The listing builds one solid part. Answer for the finished solid, in the listing's coordinates (mm). Give positions to 0.01 mm unless a question says otherwise; leave off trailing zeros. Order: outer loops, then holes, each group sorted by start corner. A loop starts at its lowest first (then second) coordinate and runs counter-clockwise, first axis right, second up. Notation, with made-up numbers: (50.5, 7) -> (95.5, 7) arc R25 ccw to (95.5, 38) -> close; hole circle Ø1 at (-16.5, 84). An arc over 180 degrees is marked (long way). Answer as a JSON object with one key per item and string values. Group by question number.
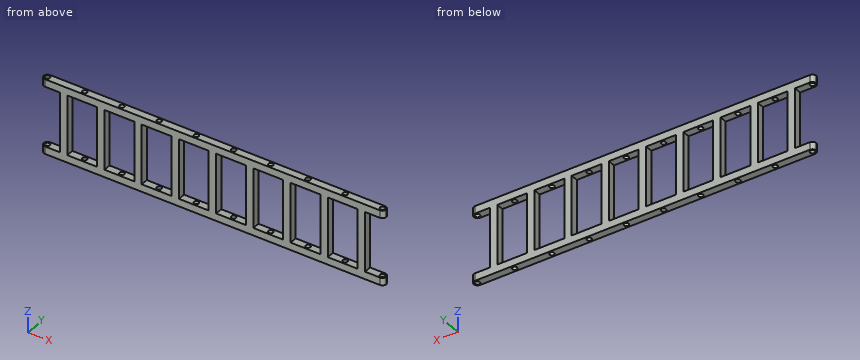
```python
from build123d import *

# Parameters (mm, degrees)
SKETCH1_W           = 25.4
SKETCH1_H           = 50.8
BOSS_EXTRUDE1_DEPTH = 6.35
CUT_EXTRUDE1_REACH  = 161.384
SKETCH2_R           = 1.9939
FILLET2_R           = 3.175


with BuildPart() as part:
    # Sketch1 → Boss-Extrude1 (new body)
    with BuildSketch(Plane(origin=(0, 0, 0), x_dir=(1, 0, 0), z_dir=(0, 1, 0))):
        Polygon((-146.05, 25.4), (-130.175, 25.4), (-130.175, -25.4), (-146.05, -25.4), (-146.05, -31.75), (146.05, -31.75), (146.05, -25.4), (130.175, -25.4), (130.175, 25.4), (146.05, 25.4), (146.05, 31.75), (-146.05, 31.75), align=None)
        with Locations((-15.875, 0)):
            Rectangle(SKETCH1_W, SKETCH1_H, mode=Mode.SUBTRACT)
        with Locations((111.125, 0)):
            Rectangle(SKETCH1_W, SKETCH1_H, mode=Mode.SUBTRACT)
        with Locations((-47.625, 0)):
            Rectangle(SKETCH1_W, SKETCH1_H, mode=Mode.SUBTRACT)
        with Locations((-79.375, 0)):
            Rectangle(SKETCH1_W, SKETCH1_H, mode=Mode.SUBTRACT)
        with Locations((-111.125, 0)):
            Rectangle(SKETCH1_W, SKETCH1_H, mode=Mode.SUBTRACT)
        with Locations((79.375, 0)):
            Rectangle(SKETCH1_W, SKETCH1_H, mode=Mode.SUBTRACT)
        with Locations((47.625, 0)):
            Rectangle(SKETCH1_W, SKETCH1_H, mode=Mode.SUBTRACT)
        with Locations((15.875, 0)):
            Rectangle(SKETCH1_W, SKETCH1_H, mode=Mode.SUBTRACT)
    extrude(amount=-BOSS_EXTRUDE1_DEPTH)

    # Cut-Extrude1: up to this face of the body (flat: up to its plane)
    cut_extrude1_end = Plane(part.part.faces().sort_by_distance((0, -3.175, -31.75))[0])
    # Sketch2 → Cut-Extrude1 (cut, up to the picked face)
    with BuildSketch(Plane.XY.offset(31.75), mode=Mode.PRIVATE) as cut_extrude1_sk1:
        with Locations((-142.875, -3.175)):
            Circle(SKETCH2_R)
    cut_extrude1_tool1 = split(extrude(cut_extrude1_sk1.sketch, amount=-CUT_EXTRUDE1_REACH, mode=Mode.PRIVATE), bisect_by=cut_extrude1_end, keep=Keep.BOTH, mode=Mode.PRIVATE)
    # Sketch2 → Cut-Extrude1 (cut, up to the picked face)
    with BuildSketch(Plane.XY.offset(31.75), mode=Mode.PRIVATE) as cut_extrude1_sk2:
        with Locations((-111.125, -3.175)):
            Circle(SKETCH2_R)
    cut_extrude1_tool2 = split(extrude(cut_extrude1_sk2.sketch, amount=-CUT_EXTRUDE1_REACH, mode=Mode.PRIVATE), bisect_by=cut_extrude1_end, keep=Keep.BOTH, mode=Mode.PRIVATE)
    # Sketch2 → Cut-Extrude1 (cut, up to the picked face)
    with BuildSketch(Plane.XY.offset(31.75), mode=Mode.PRIVATE) as cut_extrude1_sk3:
        with Locations((-79.375, -3.175)):
            Circle(SKETCH2_R)
    cut_extrude1_tool3 = split(extrude(cut_extrude1_sk3.sketch, amount=-CUT_EXTRUDE1_REACH, mode=Mode.PRIVATE), bisect_by=cut_extrude1_end, keep=Keep.BOTH, mode=Mode.PRIVATE)
    # Sketch2 → Cut-Extrude1 (cut, up to the picked face)
    with BuildSketch(Plane.XY.offset(31.75), mode=Mode.PRIVATE) as cut_extrude1_sk4:
        with Locations((-47.625, -3.175)):
            Circle(SKETCH2_R)
    cut_extrude1_tool4 = split(extrude(cut_extrude1_sk4.sketch, amount=-CUT_EXTRUDE1_REACH, mode=Mode.PRIVATE), bisect_by=cut_extrude1_end, keep=Keep.BOTH, mode=Mode.PRIVATE)
    # Sketch2 → Cut-Extrude1 (cut, up to the picked face)
    with BuildSketch(Plane.XY.offset(31.75), mode=Mode.PRIVATE) as cut_extrude1_sk5:
        with Locations((-15.875, -3.175)):
            Circle(SKETCH2_R)
    cut_extrude1_tool5 = split(extrude(cut_extrude1_sk5.sketch, amount=-CUT_EXTRUDE1_REACH, mode=Mode.PRIVATE), bisect_by=cut_extrude1_end, keep=Keep.BOTH, mode=Mode.PRIVATE)
    # Sketch2 → Cut-Extrude1 (cut, up to the picked face)
    with BuildSketch(Plane.XY.offset(31.75), mode=Mode.PRIVATE) as cut_extrude1_sk6:
        with Locations((15.875, -3.175)):
            Circle(SKETCH2_R)
    cut_extrude1_tool6 = split(extrude(cut_extrude1_sk6.sketch, amount=-CUT_EXTRUDE1_REACH, mode=Mode.PRIVATE), bisect_by=cut_extrude1_end, keep=Keep.BOTH, mode=Mode.PRIVATE)
    # Sketch2 → Cut-Extrude1 (cut, up to the picked face)
    with BuildSketch(Plane.XY.offset(31.75), mode=Mode.PRIVATE) as cut_extrude1_sk7:
        with Locations((47.625, -3.175)):
            Circle(SKETCH2_R)
    cut_extrude1_tool7 = split(extrude(cut_extrude1_sk7.sketch, amount=-CUT_EXTRUDE1_REACH, mode=Mode.PRIVATE), bisect_by=cut_extrude1_end, keep=Keep.BOTH, mode=Mode.PRIVATE)
    # Sketch2 → Cut-Extrude1 (cut, up to the picked face)
    with BuildSketch(Plane.XY.offset(31.75), mode=Mode.PRIVATE) as cut_extrude1_sk8:
        with Locations((79.375, -3.175)):
            Circle(SKETCH2_R)
    cut_extrude1_tool8 = split(extrude(cut_extrude1_sk8.sketch, amount=-CUT_EXTRUDE1_REACH, mode=Mode.PRIVATE), bisect_by=cut_extrude1_end, keep=Keep.BOTH, mode=Mode.PRIVATE)
    # Sketch2 → Cut-Extrude1 (cut, up to the picked face)
    with BuildSketch(Plane.XY.offset(31.75), mode=Mode.PRIVATE) as cut_extrude1_sk9:
        with Locations((111.125, -3.175)):
            Circle(SKETCH2_R)
    cut_extrude1_tool9 = split(extrude(cut_extrude1_sk9.sketch, amount=-CUT_EXTRUDE1_REACH, mode=Mode.PRIVATE), bisect_by=cut_extrude1_end, keep=Keep.BOTH, mode=Mode.PRIVATE)
    # Sketch2 → Cut-Extrude1 (cut, up to the picked face)
    with BuildSketch(Plane.XY.offset(31.75), mode=Mode.PRIVATE) as cut_extrude1_sk10:
        with Locations((142.875, -3.175)):
            Circle(SKETCH2_R)
    cut_extrude1_tool10 = split(extrude(cut_extrude1_sk10.sketch, amount=-CUT_EXTRUDE1_REACH, mode=Mode.PRIVATE), bisect_by=cut_extrude1_end, keep=Keep.BOTH, mode=Mode.PRIVATE)
    add(cut_extrude1_tool1.solids().sort_by(Axis((-142.875, -3.175, 31.75), (0, 0, -1)))[0], mode=Mode.SUBTRACT)
    add(cut_extrude1_tool2.solids().sort_by(Axis((-111.125, -3.175, 31.75), (0, 0, -1)))[0], mode=Mode.SUBTRACT)
    add(cut_extrude1_tool3.solids().sort_by(Axis((-79.375, -3.175, 31.75), (0, 0, -1)))[0], mode=Mode.SUBTRACT)
    add(cut_extrude1_tool4.solids().sort_by(Axis((-47.625, -3.175, 31.75), (0, 0, -1)))[0], mode=Mode.SUBTRACT)
    add(cut_extrude1_tool5.solids().sort_by(Axis((-15.875, -3.175, 31.75), (0, 0, -1)))[0], mode=Mode.SUBTRACT)
    add(cut_extrude1_tool6.solids().sort_by(Axis((15.875, -3.175, 31.75), (0, 0, -1)))[0], mode=Mode.SUBTRACT)
    add(cut_extrude1_tool7.solids().sort_by(Axis((47.625, -3.175, 31.75), (0, 0, -1)))[0], mode=Mode.SUBTRACT)
    add(cut_extrude1_tool8.solids().sort_by(Axis((79.375, -3.175, 31.75), (0, 0, -1)))[0], mode=Mode.SUBTRACT)
    add(cut_extrude1_tool9.solids().sort_by(Axis((111.125, -3.175, 31.75), (0, 0, -1)))[0], mode=Mode.SUBTRACT)
    add(cut_extrude1_tool10.solids().sort_by(Axis((142.875, -3.175, 31.75), (0, 0, -1)))[0], mode=Mode.SUBTRACT)

    # Fillet2
    fillet2_edges = [part.edges().sort_by_distance(p)[0] for p in [
        (-146.05, -6.35, 28.575),
        (-146.05, 0, 28.575),
        (-146.05, -6.35, -28.575),
        (-146.05, 0, -28.575),
        (146.05, -6.35, -28.575),
        (146.05, 0, -28.575),
        (146.05, -6.35, 28.575),
        (146.05, 0, 28.575),
    ]]
    fillet(fillet2_edges, radius=FILLET2_R - 0.0001)  # a hair under: the kernel refuses the full size


solid = part.part
```
(1) Find the intervals of material crossed by line 1 along Z through (x, y) = (-52.5, -1); line 2 along X through (y, z) = (-5.5, -27), in increasing order. Write a range as [from, to].
(2) A cutting plane is placed at B-B (z = -28). State how many separate pieces and enclosed holes the cut face has, and give its area (3 significant figures).
(3) A cutting plane is placed at A-A (x = 86.5). Determine the outline of the cut face in (y, z).
(4) Flat-ended cylindrical pins translate along their axes: pin 1 Ø3 at (y, z) = (-2, -5.5) entering from -X (3 decimals); pin 2 Ø1.5 at (y, z) = (-1, -20) entering from +X (3 decimals). Find the tip coordinate at first contact, or state that the pin passes through.
Check sheet entries:
{
 "1": {"line 1": "z = [-31.75, -25.4], [25.4, 31.75]", "line 2": "x = [-145.04, 145.04]"},
 "2": {"separate pieces": "1", "enclosed holes": "10", "area": "1,720 mm2"},
 "3": {"outline": "(-6.35, -31.75) -> (0, -31.75) -> (0, -25.4) -> (-6.35, -25.4) -> close; (-6.35, 25.4) -> (0, 25.4) -> (0, 31.75) -> (-6.35, 31.75) -> close"},
 "4": {"pin 1": "stops at x = -130.175", "pin 2": "stops at x = 130.175"}
}
